```python
from build123d import *

# Parameters (mm, degrees)
BOSS_EXTRUDE1_DEPTH = 40
SKETCH3_R           = 8.5
BOSS_EXTRUDE2_DEPTH = 8
SKETCH4_R           = 14
BOSS_EXTRUDE3_DEPTH = 6
SKETCH13_R          = 1.25
CUT_EXTRUDE8_DEPTH  = 3
SKETCH14_R          = 5.25
CUT_EXTRUDE9_DEPTH  = 6
SKETCH15_R          = 2.25
CUT_EXTRUDE10_DEPTH = 4.5


with BuildPart() as part:
    # Sketch1 → Boss-Extrude1 (new body)
    with BuildSketch(Plane(origin=(0, 0, 0), x_dir=(1, 0, 0), z_dir=(0, 1, 0))):
        Polygon((-4.807996979, 0), (-2.40399849, -4.163847525), (2.40399849, -4.163847525), (4.807996979, 0), (2.40399849, 4.163847525), (-2.40399849, 4.163847525), align=None)
    extrude(amount=BOSS_EXTRUDE1_DEPTH)

    # Sketch3 → Boss-Extrude2 (add)
    with BuildSketch(Plane(origin=(0, 0, 0), x_dir=(-1, 0, 0), z_dir=(0, -1, 0))):
        Circle(SKETCH3_R)
    extrude(amount=BOSS_EXTRUDE2_DEPTH)

    # Sketch4 → Boss-Extrude3 (add)
    with BuildSketch(Plane(origin=(0, -8, 0), x_dir=(-1, 0, 0), z_dir=(0, -1, 0))):
        Circle(SKETCH4_R)
    extrude(amount=BOSS_EXTRUDE3_DEPTH)

    # Sketch13 → Cut-Extrude8 (cut)
    with BuildSketch(Plane(origin=(0, -14, 0), x_dir=(-1, 0, 0), z_dir=(0, -1, 0))):
        with Locations((7.588295109, 7.963527946)):
            Circle(SKETCH13_R)
        with Locations((10.996799542, 0.265329684)):
            Circle(SKETCH13_R)
        with Locations((7.963527946, -7.588295109)):
            Circle(SKETCH13_R)
        with Locations((0.265329684, -10.996799542)):
            Circle(SKETCH13_R)
        with Locations((-7.588295109, -7.963527946)):
            Circle(SKETCH13_R)
        with Locations((-10.996799542, -0.265329684)):
            Circle(SKETCH13_R)
        with Locations((-7.963527946, 7.588295109)):
            Circle(SKETCH13_R)
        with Locations((-0.265329684, 10.996799542)):
            Circle(SKETCH13_R)
    extrude(amount=-CUT_EXTRUDE8_DEPTH, mode=Mode.SUBTRACT)

    # Sketch14 → Cut-Extrude9 (cut)
    with BuildSketch(Plane(origin=(0, -14, 0), x_dir=(-1, 0, 0), z_dir=(0, -1, 0))):
        Circle(SKETCH14_R)
    extrude(amount=-CUT_EXTRUDE9_DEPTH, mode=Mode.SUBTRACT)

    # Sketch15 → Cut-Extrude10 (cut)
    with BuildSketch(Plane(origin=(0, -8, 0), x_dir=(1, 0, 0), z_dir=(0, 1, 0))):
        with Locations((10.996799542, -0.265329684)):
            Circle(SKETCH15_R)
        with Locations((7.588295109, -7.963527946)):
            Circle(SKETCH15_R)
        with Locations((-0.265329684, -10.996799542)):
            Circle(SKETCH15_R)
        with Locations((-7.963527946, -7.588295109)):
            Circle(SKETCH15_R)
        with Locations((-10.996799542, 0.265329684)):
            Circle(SKETCH15_R)
        with Locations((-7.588295109, 7.963527946)):
            Circle(SKETCH15_R)
        with Locations((0.265329684, 10.996799542)):
            Circle(SKETCH15_R)
        with Locations((7.963527946, 7.588295109)):
            Circle(SKETCH15_R)
    extrude(amount=-CUT_EXTRUDE10_DEPTH, mode=Mode.SUBTRACT)


solid = part.part
```
Work out the finished part from the listing and answer in its coordinate system (mm). A direction names the side the tool comes from. Round coordinates to 2 decimals unless told otherwise and drop trailing zeros. Write each loop counter-clockwise with the first axis right and the second up, starting at its lowest first coordinate (ties: lowest second). Pieces come first, ordered by that corner, then holes.
1) Consider probe 1 along Y at (x, z) = (1.25, 9.25); probe 2 along Y at (x, z) = (-4.25, 4.75); probe 3 along X at (y, z) = (-10.5, -4.75). Determine where each line is inside the solid, lowest interval first.
2) A cutting plane is placed at C-C on x = -11.5. Determine the outline of the cut face in (y, z), and give its area (3 significant figures).
3) A cutting plane is placed at A-A on x = 0. Give the number of separate pieces and of enclosed holes in the cut face, and give its area (3 significant figures).
4) A cutting plane is placed at D-D on x = 3.25. Determine the outline of the cut face in (y, z), and give its area (3 significant figures).
5) Flat-ended cylindrical pins translate along their axes: P1, Ø6, axis at x = -4.5, y = 23, coming from the -Z side; P2, Ø2, axis at x = -8, z = 6.5, coming from the +Y side; P3, Ø3.5, axis at x = 10.5, z = 0, coming from the +Y side; P4, Ø8, axis at x = 9, y = 20.5, coming from the +Z side. Find the tip coordinate at first contact, or state that the pin passes through.
6) A cutting plane is placed at B-B on y = 20.5. Determine the outline of the cut face in (x, z), and give its area (3 significant figures).
7) Which of the six approach directions +Z, -Z, +X, -X, +Y, -Y give full straight-line access (tool end or side, diameter ignored) to faces 1 (the face through (-3.59, 19.72, -2.11)), 2 (the face through (-5, -11, -1.6)), 3 (the face through (-8.85, -10.22, -0.94))?
8) Determine the mould class of faces 4 (the face through (-4.57, -3.944, -7.167)), 5 (the face through (0, -14, 6)), 6 (the face through (1, -12.5, 12)), 7 (the face through (0, 20, 4.164)) for opening direction Z: pulls with the +Z half, pulls with the -Z half, needs draft (parallel to the pull), parting line crosses it, or undercut.
Entries:
1. probe 1: y = -14 to -8
1. probe 2: y = -14 to 0
1. probe 3: x = -13.17 to -2.24, 2.24 to 13.17
2. outline: (-14, -7.98) - (-8, -7.98) - (-8, -2.46) - (-12.5, -2.46) - (-12.5, -1.41) - (-14, -1.41) - close; (-14, 0.88) - (-12.5, 0.88) - (-12.5, 1.93) - (-8, 1.93) - (-8, 7.98) - (-14, 7.98) - close
2. area: 72.6 mm2
3. separate pieces: 3
3. enclosed holes: 0
3. area: 527 mm2
4. outline: (-14, -13.62) - (-8, -13.62) - (-8, -7.85) - (0, -7.85) - (0, -2.7) - (40, -2.7) - (40, 2.7) - (0, 2.7) - (0, 7.85) - (-8, 7.85) - (-8, 13.62) - (-14, 13.62) - (-14, 4.12) - (-8, 4.12) - (-8, -4.12) - (-14, -4.12) - close
4. area: 455 mm2
5. P1: stops at z = -4.16
5. P2: stops at y = -12.5
5. P3: stops at y = -8
5. P4: passes through
6. outline: (-4.81, 0) - (-2.4, -4.16) - (2.4, -4.16) - (4.81, 0) - (2.4, 4.16) - (-2.4, 4.16) - close
6. area: 60.1 mm2
7. face 1: -Z, -X, +Y
7. face 2: -Y
7. face 3: +Y
8. face 4: parting line crosses it
8. face 5: needs draft
8. face 6: undercut
8. face 7: pulls with the +Z half
